Can you work these out from the drawing? Everything is in mm from the part's minimum corner. Round coordinates to 2 decimals unless told otherwise and drop trailing zeros. Loops run counter-clockwise (first coordinate to the right, second up) from the corner with the lowest first, then second, coordinate; pieces in that order, holes last. Notation, with made-up numbers: M 39,3 L 79,3 A10 cw 79,16 Z; hole C 46,-21.5 d1. An arc over 180 degrees is marked long. Use a Markdown table: item, result.
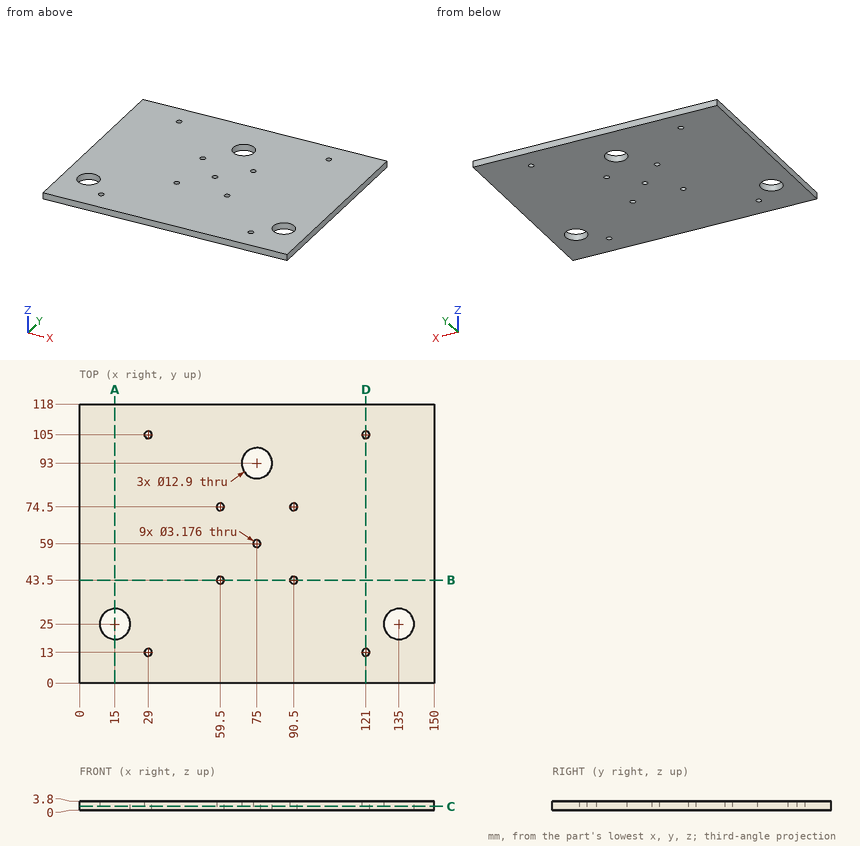
Q1. Imagine slicing it at D-D, the plane x = 121. Please give me the cut outline in (y, z).
Return value:
| item | result |
|---|---|
| outline | M 0,0 L 11.41,0 L 11.41,3.8 L 0,3.8 Z; M 14.59,0 L 103.41,0 L 103.41,3.8 L 14.59,3.8 Z; M 106.59,0 L 118,0 L 118,3.8 L 106.59,3.8 Z |
Q2. I need wall thicknesses on line 1 (Y direction, x = 29, z = 2.7); line 2 (X direction, y = 74.5, z = 2.5); line 3 (X direction, y = 105, z = 1.9). Which ranges of each line are inside material? Lowest first, please. Write a range as from..to.
Return value:
| item | result |
|---|---|
| line 1 | y = 0..11.41, 14.59..103.41, 106.59..118 |
| line 2 | x = 0..57.91, 61.09..88.91, 92.09..150 |
| line 3 | x = 0..27.41, 30.59..119.41, 122.59..150 |
Q3. Imagine slicing it at B-B, the plane y = 43.5. Please give me the cut outline in (x, z).
Return value:
| item | result |
|---|---|
| outline | M 0,0 L 57.91,0 L 57.91,3.8 L 0,3.8 Z; M 61.09,0 L 88.91,0 L 88.91,3.8 L 61.09,3.8 Z; M 92.09,0 L 150,0 L 150,3.8 L 92.09,3.8 Z |
Q4. Imagine slicing it at C-C, the plane z = 1.55. Give the number of separate pieces and of enclosed holes in the cut face, then the cut area to 3 significant figures.
Return value:
| item | result |
|---|---|
| separate pieces | 1 |
| enclosed holes | 12 |
| area | 17,200 mm^2 |
Q5. Imagine slicing it at A-A, the plane x = 15. Please give me the cut outline in (y, z), then the cut area to 3 significant figures.
Return value:
| item | result |
|---|---|
| outline | M 0,0 L 18.55,0 L 18.55,3.8 L 0,3.8 Z; M 31.45,0 L 118,0 L 118,3.8 L 31.45,3.8 Z |
| area | 399 mm^2 |
